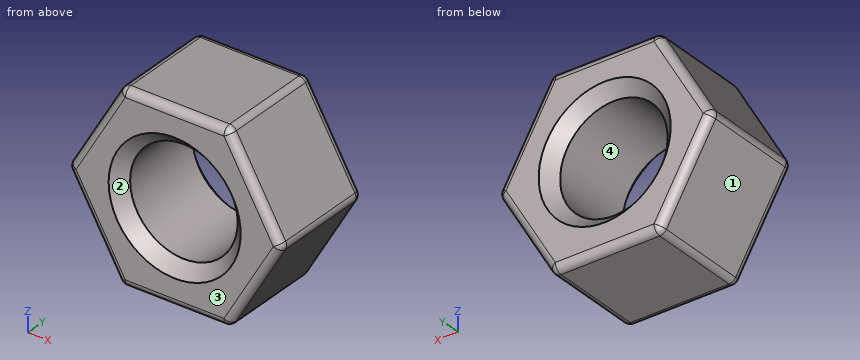
Autodesk Inventor part; units mm, degrees
ref_plane "YZ Plane" through (0, 0, 0) normal (1, 0, 0) x (0, 1, 0)
ref_plane "XZ Plane" through (0, 0, 0) normal (0, 1, 0) x (-1, 0, 0)
ref_plane "XY Plane" through (0, 0, 0) normal (0, 0, 1) x (1, 0, 0)
sketch "Boceto1" plane through (0, 0, 0) normal (0, 1, 0) x (-1, 0, 0)
  line L0 (-5.5852, -5.9648) -> (1.4148, -5.9648)
  line L1 (1.4148, -5.9648) -> (4.9148, 0.0974)
  line L2 (4.9148, 0.0974) -> (1.4148, 6.1595)
  line L3 (1.4148, 6.1595) -> (-5.5852, 6.1595)
  line L4 (-5.5852, 6.1595) -> (-9.0852, 0.0974)
  line L5 (-9.0852, 0.0974) -> (-5.5852, -5.9648)
  circle A0 centre (-2.0852, 0.0974) radius 3.5
  dimension "d21" = 7
  dimension "d22" = 7
  dimension "d23" = 120
  dimension "d24" = 7
  dimension "d25" = 7
  dimension "d26" = 7
  dimension "d27" = 120
  dimension "d28" = 7
extrude "Extrusión1" add sketch "Boceto1" along normal blind 7
thread "Rosca1"
fillet "Empalme1" radius 0.5 18 edges at (-1.4148, 3.5, 6.1595) (-4.9148, 3.5, 0.0974) (-1.4148, 3.5, -5.9648) (5.5852, 3.5, -5.9648) (9.0852, 3.5, 0.0974) (5.5852, 3.5, 6.1595) (7.3352, 0, 3.1284) (2.0852, 0, 6.1595) (-3.1648, 0, 3.1284) (-3.1648, 0, -2.9337) (2.0852, 0, -5.9648) (7.3352, 0, -2.9337) (7.3352, 7, 3.1284) (7.3352, 7, -2.9337) (2.0852, 7, -5.9648) (-3.1648, 7, -2.9337) (-3.1648, 7, 3.1284) (2.0852, 7, 6.1595)
chamfer "Chaflán1" distance 0.8 angle 45 2 edges at (5.5852, 7, 0.0974) (5.5852, 0, 0.0974)
thread "Rosca2"
thread "Rosca3"
properties material "Acero"
Input: part model. Units: mm. Frame: model coordinates. Face numbers are marked on the shaded views. Give positions to 0.01 mm unless a question says otherwise; leave off trailing zeros. Order: outer loops, then holes, each group sorted by start corner. A loop starts at its lowest first (then second) coordinate and runs counter-clockwise, first axis right, second up.
1. Pin query (flat end, axial travel): pin 1 (1.5 mm diameter, centred on x = 3, z = -0.5, fed in from -Y). Return the tip coordinate at first contact, or that it passes through.
Derived:
pin 1: passes through
2. Mould query, pull axis X, two halves, no side actions, for the marked faces 1, 2, 3 and 4. Classes: released by +X, released by -X, zero draft, split by the parting line, or undercut.
Derived:
face 1: released by -X
face 2: undercut
face 3: zero draft
face 4: undercut
3. Section A-A on y = 6. Return the cut outline in (x, z), and give its area (3 significant figures).
Derived:
outline: (-4.77, -0.15) - (-1.56, -5.71) arc R0.5 ccw to (-1.13, -5.96) - (5.3, -5.96) arc R0.5 ccw to (5.73, -5.71) - (8.94, -0.15) arc R0.5 ccw to (8.94, 0.35) - (5.73, 5.91) arc R0.5 ccw to (5.3, 6.16) - (-1.13, 6.16) arc R0.5 ccw to (-1.56, 5.91) - (-4.77, 0.35) arc R0.5 ccw to start; hole circle Ø7 at (2.09, 0.1)
area: 88.7 mm2
4. Material intervals for L1, parallel to Z at x = 0.25, y = 3.75; L2, parallel to Z at x = 3.75, y = 5.5; L3, parallel to X at y = 1.5, z = -1.5, sorted ascending.
Derived:
L1: z = -5.96 to -2.88, 3.08 to 6.16
L2: z = -5.96 to -2.98, 3.18 to 6.16
L3: x = -3.99 to -1.03, 5.2 to 8.16
